from build123d import *

# Parameters (mm, degrees)
STOCK_NOZZLE4_1_OUTLINE_W = 4.964466094
STOCK_NOZZLE4_1_OUTLINE_H = 15
STOCK_NOZZLE4_1_DEPTH     = 50
STOCK_NOZZLE4_1_START     = 20
STOCK_NOZZLE4_1_2_DEPTH   = 30
SKETCH1_W                 = 20
SKETCH1_H                 = 2
CUT_EXTRUDE1_DEPTH        = 80.180046713
SKETCH2_W                 = 11.16019391
SKETCH2_H                 = 20
CUT_EXTRUDE2_DEPTH        = 79.825629065
SKETCH6_R                 = 1.3
CUT_EXTRUDE3_DEPTH        = 79.825629065
SKETCH7_W                 = 1.8
SKETCH7_H                 = 4.2
CUT_EXTRUDE4_DEPTH        = 4.964466094
SKETCH8_R                 = 3.75
CUT_EXTRUDE5_DEPTH        = 2


# Read off the part's stored shape, not the designer's step: Stock-nozzle4-1
with BuildPart() as part:
    # Stock-nozzle4-1 outline → Stock-nozzle4-1 (new body)
    with BuildSketch(Plane(origin=(0, 0, 0), x_dir=(1, 0, 0), z_dir=(0, 1, 0))):
        with Locations((53.517766953, -7.5)):
            Rectangle(STOCK_NOZZLE4_1_OUTLINE_W, STOCK_NOZZLE4_1_OUTLINE_H)
    extrude(amount=STOCK_NOZZLE4_1_DEPTH)

    # Stock-nozzle4-1 2 outline → Stock-nozzle4-1 2 (add)
    with BuildSketch(Plane(origin=(0, 0, 0), x_dir=(1, 0, 0), z_dir=(0, 1, 0)).offset(STOCK_NOZZLE4_1_START)):
        Polygon((56, -11.035533906), (56, -15), (59.535533906, -15), (59.535533906, -7.5), align=None)
    extrude(amount=STOCK_NOZZLE4_1_2_DEPTH)

    # Sketch1 → Cut-Extrude1 (cut, through all)
    with BuildSketch(Plane(origin=(0, 50, 0), x_dir=(1, 0, 0), z_dir=(0, 1, 0))):
        with Locations((59.035533906, -14)):
            Rectangle(SKETCH1_W, SKETCH1_H)
    extrude(amount=-CUT_EXTRUDE1_DEPTH, mode=Mode.SUBTRACT)

    # Sketch2 → Cut-Extrude2 (cut, through all)
    with BuildSketch(Plane.XY.offset(13)):
        with Locations((56.580096955, 10)):
            Rectangle(SKETCH2_W, SKETCH2_H)
    extrude(amount=-CUT_EXTRUDE2_DEPTH, mode=Mode.SUBTRACT)

    # Sketch6 → Cut-Extrude3 (cut, through all)
    with BuildSketch(Plane.XY.offset(13)):
        with Locations((53.25, 45)):
            Circle(SKETCH6_R)
        with Locations((53.25, 25)):
            Circle(SKETCH6_R)
    extrude(amount=-CUT_EXTRUDE3_DEPTH, mode=Mode.SUBTRACT)

    # Sketch7 → Cut-Extrude4 (cut)
    with BuildSketch(Plane.ZY.offset(-51.035533906)):
        with Locations((5.9, 44.8)):
            Rectangle(SKETCH7_W, SKETCH7_H)
        with Locations((5.9, 24.8)):
            Rectangle(SKETCH7_W, SKETCH7_H)
    extrude(amount=-CUT_EXTRUDE4_DEPTH, mode=Mode.SUBTRACT)

    # Sketch8 → Cut-Extrude5 (cut)
    with BuildSketch(Plane(origin=(0, 0, 0), x_dir=(-1, 0, 0), z_dir=(0, 0, -1))):
        with Locations((-48.435533906, 30.5)):
            Circle(SKETCH8_R)
    extrude(amount=-CUT_EXTRUDE5_DEPTH, mode=Mode.SUBTRACT)


solid = part.part
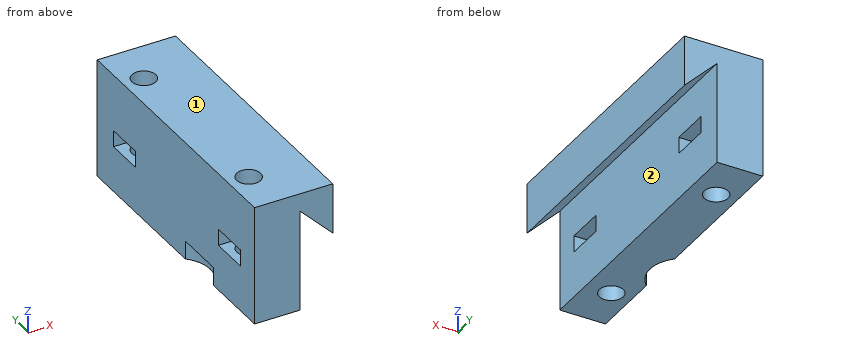
Can you work these out from the model? Positions are in its coordinate system, mm. Face numbers are marked on the shaded views. A direction names the side the tool comes from. Round coordinates to 2 decimals unless told otherwise and drop trailing zeros. Loops run counter-clockwise (first coordinate to the right, second up) from the corner with the lowest first, then second, coordinate; pieces in that order, holes last. Notation, with made-up numbers: (71, 10.25) - (94, 10.25) arc R13 cw to (94, 21.25) - close; hole circle Ø11 at (86.5, -13.75). An arc over 180 degrees is marked (long way). Write item = value, one per line. Start each with the question number.
(1) If I drill on probe 1 along Y at (x, z) = (53.25, 8.5); probe 2 along Y at (x, z) = (52, 5.75); probe 3 along Z at (x, y) = (53.25, 43.5), over which ranges is the centre line in solid material (lowest first)? Write a range as [from, to].
(2) For the marked faces 1 and 2, which set-ups out of +Z, -Z, +X, -X, +Y, -Y let a thin tool reach every point of the face, with its end or its side?
(3) If we section it at A-A (y = 25): Please give me the cut outline in (x, z).
(4) If we section it at D-D (x = 53.25): Please give me the cut outline in (y, z).
(5) If we section it at B-B (z = 6.5): Please give me the cut outline in (x, y), and give its area (3 significant figures).
(6) If we section it at C-C (z = 10.75): Please give me the cut outline in (x, y), and give its area (3 significant figures).
(7) For P1, Ø1.6, axis at x = 53.25, y = 45, coming from the -Z side; P2, Ø3.5, axis at x = 53.25, y = 25, coming from the +Z side, each with a flat end and sliding along its axis, tell me the tip position at first contact or that it passes through.
Ans:
q1.probe_1 = [20, 23.7], [26.3, 43.7], [46.3, 50]
q1.probe_2 = [20, 22.7], [26.9, 42.7], [46.9, 50]
q1.probe_3 = [0, 5], [6.8, 13]
q2.face_1 = +Z, +X, -X, +Y, -Y
q2.face_2 = -Z, +Y, -Y
q3.outline = (51.04, 0) - (51.95, 0) - (51.95, 5) - (51.04, 5) - close; (51.04, 6.8) - (51.95, 6.8) - (51.95, 13) - (51.04, 13) - close; (54.55, 0) - (56, 0) - (56, 5) - (54.55, 5) - close; (54.55, 6.8) - (56, 6.8) - (56, 11.04) - (59.54, 7.5) - (59.54, 13) - (54.55, 13) - close
q4.outline = (20, 0) - (23.7, 0) - (23.7, 5) - (22.7, 5) - (22.7, 6.8) - (23.7, 6.8) - (23.7, 13) - (20, 13) - close; (26.3, 0) - (43.7, 0) - (43.7, 5) - (42.7, 5) - (42.7, 6.8) - (43.7, 6.8) - (43.7, 13) - (26.3, 13) - (26.3, 6.8) - (26.9, 6.8) - (26.9, 5) - (26.3, 5) - close; (46.3, 0) - (50, 0) - (50, 13) - (46.3, 13) - (46.3, 6.8) - (46.9, 6.8) - (46.9, 5) - (46.3, 5) - close
q5.outline = (51.04, 20) - (56, 20) - (56, 22.7) - (51.04, 22.7) - close; (51.04, 26.9) - (56, 26.9) - (56, 42.7) - (51.04, 42.7) - close; (51.04, 46.9) - (56, 46.9) - (56, 50) - (51.04, 50) - close
q5.area = 107 mm²
q6.outline = (51.04, 20) - (56, 20) - (56, 50) - (51.04, 50) - close; (56.29, 20) - (59.54, 20) - (59.54, 50) - (56.29, 50) - close; hole circle Ø2.6 at (53.25, 25); hole circle Ø2.6 at (53.25, 45)
q6.area = 236 mm²
q7.P1 = through
q7.P2 = 13
